Source: CAD feature listing. Evaluate the final solid. Frame: model axes, mm. Coordinates: 2 decimals unless noted, no trailing zeros. Write each loop counter-clockwise with the first axis right and the second up, starting at its lowest first coordinate (ties: lowest second). Pieces come first, ordered by that corner, then holes. Notation, with made-up numbers: M -23.75,42 L -1.75,42 A22 cw -1.75,62 Z; hole C 0,-32 d8. An arc over 180 degrees is marked long. Write item = value, one per line. Start each with the question number.
1. Section query B-B (x = 13.25). Output: boundary loops of the cut face in (y, z).
2. Section query A-A (z = -139.5). Output: boundary loops of the cut face in (x, y), then the cut area to 3 significant figures.
3. Section query D-D (x = -2.25). Output: boundary loops of the cut face in (y, z).
4. Line query: line 1 along Y through (x, z) = (1, -138.25); line 2 along X through (y, z) = (-4.5, -133); line 3 along Z through (x, y) = (0, -0.25). Output: solid intervals per line, ascending.
5. Section query C-C (y = -5.5). Output: boundary loops of the cut face in (x, z).
Autodesk Inventor part; units mm, degrees
ref_plane "YZ Plane" through (0, 0, 0) normal (1, 0, 0) x (0, 1, 0)
ref_plane "XZ Plane" through (0, 0, 0) normal (0, 1, 0) x (-1, 0, 0)
ref_plane "XY Plane" through (0, 0, 0) normal (0, 0, 1) x (1, 0, 0)
ref_plane "Work Plane1" through (-6.4883, -6.1632, -131.5017) normal (0, 1, 0) x (-1, 0, 0)
sketch "Sketch1" plane through (-6.4883, -6.1632, -131.5017) normal (0, 1, 0) x (-1, 0, 0)
  line L0 (-2, -18) -> (-2, 0)
  line L1 (-2, 0) -> (-7.4816, 0)
  line L2 (-22.4693, -8.5807) -> (-7.4816, 0)
  line L3 (-6.2906, -18) -> (-22.4693, -8.5807)
  line L4 (-2, -18) -> (-6.2906, -18)
  point P0 (-6.4883, 131.5017)
extrude "Extrusion1" add sketch "Sketch1" along normal blind 8
sketch "Sketch2" plane through (0, 0, 0) normal (1, 0, 0) x (0, 1, 0)
  line L0 (-6.1632, -140.0824) -> (1.8368, -140.0824)
  circle A0 centre (-2.1632, -140.0824) radius 3
  point P0 (0, 0)
  dimension "d2" = 6
extrude "Extrusion2" cut sketch "Sketch2" along normal through all both and the other way through all
sketch "Sketch3" plane through (-6.4883, 1.8368, -131.5017) normal (0, 1, 0) x (1, 0, 0)
  line L0 (6.2906, 18) -> (2, 18)
  line L1 (17.3164, 11.5807) -> (22.4693, 8.5807)
  line L2 (2, 18) -> (22.4693, 18)
  line L3 (22.4693, 18) -> (22.4693, 8.5807)
  line L4 (22.4693, 8.5807) -> (2, 8.5807)
  line L5 (2, 8.5807) -> (2, 18)
  point P0 (6.4883, -131.5017)
extrude "Extrusion3" cut sketch "Sketch3" against normal through all
properties part number "Wire_Clossing"
Results are:
q1.outline = M -6.16,-140.08 L -5.16,-140.08 A3 cw -4.72,-138.52 L -6.16,-138.52 Z; M 0.4,-138.52 A3 cw 0.84,-140.08 L 1.84,-140.08 L 1.84,-138.52 Z
q2.outline = M -4.49,-6.16 L 14.96,-6.16 L 14.96,-5.11 L -4.49,-5.11 Z; M -4.49,0.78 L 14.96,0.78 L 14.96,1.84 L -4.49,1.84 Z
q2.area = 41.1 mm^2
q3.outline = M -6.16,-140.08 L -5.16,-140.08 A3 cw 0.84,-140.08 L 1.84,-140.08 L 1.84,-131.5 L -6.16,-131.5 Z
q4.line_1 = -6.16 to -4.54, 0.21 to 1.84
q4.line_2 = -4.49 to 3.61
q4.line_3 = -137.77 to -131.5
q5.outline = M -4.49,-140.08 L 15.98,-140.08 L 0.99,-131.5 L -4.49,-131.5 Z
